Work out the finished part from the listing and answer in its coordinate system (mm). Face numbers are marked on the shaded views. A direction names the side the tool comes from. Round coordinates to 2 decimals unless told otherwise and drop trailing zeros. Order: outer loops, then holes, each group sorted by start corner. A loop starts at its lowest first (then second) coordinate and runs counter-clockwise, first axis right, second up. Notation, with made-up numbers: (58, -17.5) - (95, -17.5) arc R21 ccw to (95, -1.5) - close; hole circle Ø1 at (48, 34). An arc over 180 degrees is marked (long way). Put each result on its own line as item: value.
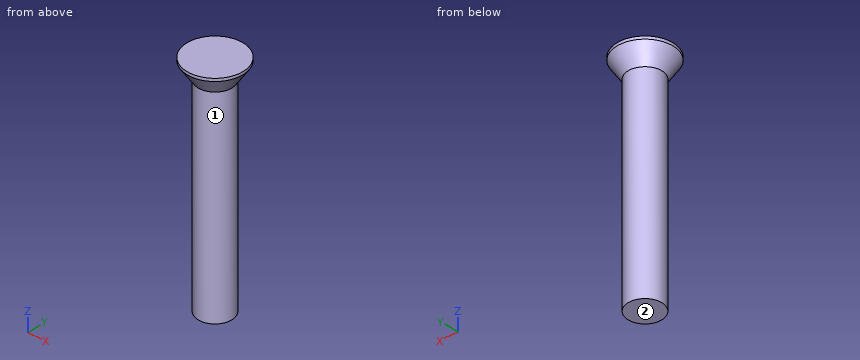
```python
from build123d import *

# Parameters (mm, degrees)
F0_R     = 5
F1_DEPTH = 3.5
F2_R     = 3
F3_DEPTH = 36.5
F4_SIZE2 = 1.99999
F4_SIZE  = 2.99999


# Not quite as in the source:
# - a fillet or chamfer is up to 0.001 mm smaller than in the source, because OpenCascade refuses the exact size


with BuildPart() as f1:
    # F0 (on Top) → F1 (new body)
    with BuildSketch(Plane.XY):
        Circle(F0_R)
    extrude(amount=F1_DEPTH)

    # F2 (on face) → F3 (join)
    with BuildSketch(Plane(origin=(0, 0, 0), x_dir=(1, 0, 0), z_dir=(0, 0, -1))):
        Circle(F2_R)
    extrude(amount=F3_DEPTH)

    # F4 (size 3 and 2 in the source; OpenCascade refuses exactly that, so slightly less here)
    f4_edges = [f1.edges().sort_by_distance(p)[0] for p in [
        (-5, 0, 0),
    ]]
    f4_side = f1.faces().sort_by_distance((-5, 0, 1.75))[0]
    chamfer(f4_edges, length=F4_SIZE, length2=F4_SIZE2, reference=f4_side)


solid = f1.part
```
1) Given pin 1 Ø1.5 at (x, z) = (-1.5, -7.5) entering from +Y; pin 2 Ø4 at (x, z) = (4, -12.5) entering from -Y; pin 3 Ø1.5 at (y, z) = (-3, -7.5) entering from +X, each flat-ended and moving along its own axis, determine where each tip first touches the part or whether it passes through.
Findings below:
pin 1: stops at y = 2.9
pin 2: stops at y = -2.24
pin 3: stops at x = 1.98
2) A cutting plane is placed at C-C on z = -6.5. Write down the section's boundary in (x, y), then the cut area to 3 significant figures.
Findings below:
outline: circle Ø6 at (0, 0)
area: 28.3 mm2
3) Straight lines are drawn through the part: L1, parallel to Y at x = 0, z = -13.5; L2, parallel to X at y = -0.5, z = -7.5; L3, parallel to Y at x = -1.5, z = -34. For each, find the intervals that lie inside material, in ascending order. Write a range as from..to.
Findings below:
L1: y = -3..3
L2: x = -2.96..2.96
L3: y = -2.6..2.6
4) A cutting plane is placed at D-D on z = 0.5. Write down the section's boundary in (x, y).
Findings below:
outline: circle Ø6.67 at (0, 0)
5) For the marked faces 1 and 2, determine the directions among +Z, -Z, +X, -X, +Y, -Y from which every point of the face is accessible in a straight line to the end or side of a thin tool.
Findings below:
face 1: -Z
face 2: -Z, +X, -X, +Y, -Y
